Part print with two shaded views. Sizes in mm from the minimum x, y, z corner. A direction names the side the tool comes from. Round coordinates to 2 decimals unless told otherwise and drop trailing zeros. Order: outer loops, then holes, each group sorted by start corner. A loop starts at its lowest first (then second) coordinate and runs counter-clockwise, first axis right, second up. Notation, with made-up numbers: (-8, 6.5) -> (10, 6.5) arc R22 ccw to (10, 13.5) -> close; hole circle Ø2 at (32, 89.25). An arc over 180 degrees is marked (long way). Put each result on its own line as item: value. Start each with the question number.
Q1. 3-axis set-ups, long thin cutter, end or side, ignore diameter. For the marked faces 1, 2 and 3: which of +Z, -Z, +X, -X, +Y, -Y reach the whole face in a straight line?
Q2. Flat gauge pins, fed straight in: P1, Ø1.5, axis at x = 6, z = 7, coming from the +Y side; P2, Ø1, axis at x = 12.7, y = 12.7, coming from the -Z side; P3, Ø1.5, axis at y = 4.5, z = 3.5, coming from the -X side (1 decimal); P4, Ø1.4, axis at x = 12.5, y = 12.5, coming from the -Z side. Where does each tip first touch, or does it go through?
Q3. Cut at C-C, the plane z = 7.75. List the corners of the cut face in (x, y).
Q4. Probe L1, parallel to Y at x = 12.7, z = 13.7 (1 decimal); L2, parallel to Y at x = 12.7, z = 0.8 (1 decimal); L3, parallel to Z at x = 22.5, y = 14.25 (1 decimal). List the from-to ranges inside material, lowest first.
Q5. Cut at B-B, the plane y = 18. List the corners of the cut face in (x, z) (1 decimal), and give its area (3 significant figures).
Q6. Cut at A-A, the plane x = 12.7. List the corners of the cut face in (y, z) (1 decimal), and give its area (3 significant figures).
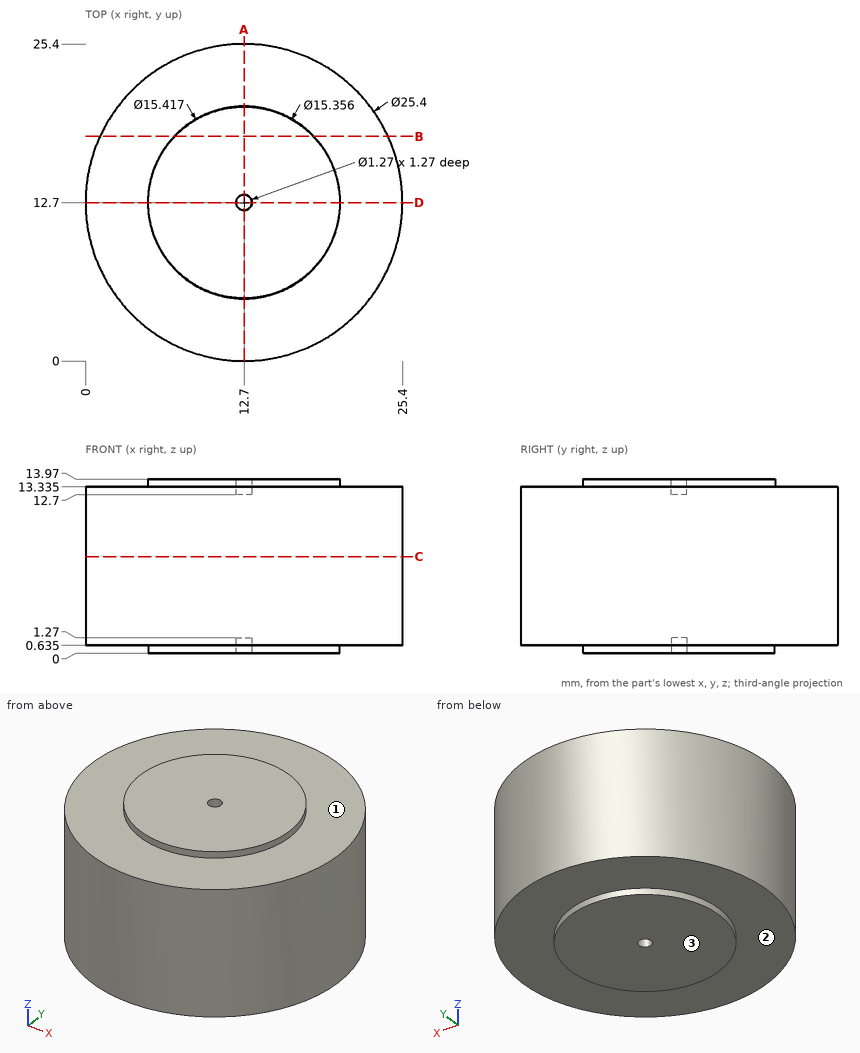
Ans:
1. face 1: +Z
1. face 2: -Z
1. face 3: -Z, +X, -X, +Y, -Y
2. P1: stops at y = 23.92
2. P2: stops at z = 1.27
2. P3: stops at x = 2.4
2. P4: stops at z = 0
3. outline: circle Ø25.4 at (12.7, 12.7)
4. L1: y = 5 to 12.1, 13.3 to 20.4
4. L2: y = 0 to 12.1, 13.3 to 25.4
4. L3: z = 0.6 to 13.3
5. outline: (1.2, 0.6) -> (7.1, 0.6) -> (7.1, 0) -> (18.3, 0) -> (18.3, 0.6) -> (24.2, 0.6) -> (24.2, 13.3) -> (18.3, 13.3) -> (18.3, 14) -> (7.1, 14) -> (7.1, 13.3) -> (1.2, 13.3) -> close
5. area: 307 mm^2
6. outline: (0, 0.6) -> (5, 0.6) -> (5, 0) -> (12.1, 0) -> (12.1, 1.3) -> (13.3, 1.3) -> (13.3, 0) -> (20.4, 0) -> (20.4, 0.6) -> (25.4, 0.6) -> (25.4, 13.3) -> (20.4, 13.3) -> (20.4, 14) -> (13.3, 14) -> (13.3, 12.7) -> (12.1, 12.7) -> (12.1, 14) -> (5, 14) -> (5, 13.3) -> (0, 13.3) -> close
6. area: 339 mm^2
